Can you work these out from the model? Positions are in its coordinate system, mm. Coordinates: 2 decimals unless noted, no trailing zeros. Order: outer loops, then holes, each group sorted by start corner. A loop starts at its lowest first (then second) coordinate and runs counter-clockwise, first axis right, second up. Notation, with made-up numbers: (45, 8.25) -> (98, 8.25) arc R15 cw to (98, 14.25) -> close; hole circle Ø10 at (-32, 18.25). An arc over 180 degrees is marked (long way). Answer in a Markdown table with one row per item.
```python
from build123d import *

# Parameters (mm, degrees)
SKETCH1_W           = 50.8
SKETCH1_H           = 95.25
SKETCH1_R           = 2.413
BOSS_EXTRUDE1_DEPTH = 6.35
FILLET1_R           = 6.35
CHAMFER1_SIZE       = 2.54


with BuildPart() as part:
    # Sketch1 → Boss-Extrude1 (new body)
    with BuildSketch(Plane.XY):
        with Locations((25.4, 47.625)):
            Rectangle(SKETCH1_W, SKETCH1_H)
        with Locations((25.4, 69.85)):
            Circle(SKETCH1_R, mode=Mode.SUBTRACT)
        with Locations((25.4, 25.4)):
            Circle(SKETCH1_R, mode=Mode.SUBTRACT)
        with Locations((25.4, 57.15)):
            Circle(SKETCH1_R, mode=Mode.SUBTRACT)
        with Locations((25.4, 12.7)):
            Circle(SKETCH1_R, mode=Mode.SUBTRACT)
        with Locations((25.4, 38.1)):
            Circle(SKETCH1_R, mode=Mode.SUBTRACT)
        with Locations((25.4, 82.55)):
            Circle(SKETCH1_R, mode=Mode.SUBTRACT)
    extrude(amount=BOSS_EXTRUDE1_DEPTH)

    # Fillet1
    fillet1_edges = [part.edges().sort_by_distance(p)[0] for p in [
        (0, 95.25, 3.175),
        (50.8, 95.25, 3.175),
        (50.8, 0, 3.175),
        (0, 0, 3.175),
    ]]
    fillet(fillet1_edges, radius=FILLET1_R)

    # Chamfer1
    chamfer1_edges = [part.edges().sort_by_distance(p)[0] for p in [
        (22.987, 69.85, 6.35),
        (22.987, 25.4, 6.35),
        (22.987, 57.15, 6.35),
        (22.987, 12.7, 6.35),
        (22.987, 38.1, 6.35),
        (22.987, 82.55, 6.35),
    ]]
    chamfer(chamfer1_edges, length=CHAMFER1_SIZE)


solid = part.part
```
(1) Suppose I cut it at A-A (z = 2). Please give me the cut outline in (x, y), and give its area (3 significant figures).
Response values:
| item | result |
|---|---|
| outline | (0, 6.35) arc R6.35 ccw to (6.35, 0) -> (44.45, 0) arc R6.35 ccw to (50.8, 6.35) -> (50.8, 88.9) arc R6.35 ccw to (44.45, 95.25) -> (6.35, 95.25) arc R6.35 ccw to (0, 88.9) -> close; hole circle Ø4.83 at (25.4, 12.7); hole circle Ø4.83 at (25.4, 25.4); hole circle Ø4.83 at (25.4, 38.1); hole circle Ø4.83 at (25.4, 57.15); hole circle Ø4.83 at (25.4, 69.85); hole circle Ø4.83 at (25.4, 82.55) |
| area | 4,690 mm2 |
(2) Suppose I cut it at B-B (y = 12.7). Please give me the cut outline in (x, z).
Response values:
| item | result |
|---|---|
| outline | (0, 0) -> (22.99, 0) -> (22.99, 3.81) -> (20.45, 6.35) -> (0, 6.35) -> close; (27.81, 0) -> (50.8, 0) -> (50.8, 6.35) -> (30.35, 6.35) -> (27.81, 3.81) -> close |
(3) We'd pull the mould along Y, two halves only. Please class faces 1 (the flat face through (25, 48, 0)), 2 (the conical face through (25.07, 59.66, 3.93)), 3 (the conical face through (26.57, 80.3, 3.933)), 4 (the cylindrical face through (48.89, 1.81, 3.22)): +Y half, -Y half, draft (parallel to the pull), parting line (faces both ways), or undercut.
Response values:
| item | result |
|---|---|
| face 1 | draft |
| face 2 | undercut |
| face 3 | undercut |
| face 4 | -Y half |
(4) Will these pins go through, and if not, where does the flat tip stop? pin 1 Ø1.5 at (x, y) = (29, 23.5) entering from +Z; pin 2 Ø6.5 at (x, y) = (25.4, 12.7) entering from +Z.
Response values:
| item | result |
|---|---|
| pin 1 | z = 6.22 |
| pin 2 | z = 4.65 |
(5) Suppose I cut it at C-C (x = 25.4). Count the separate pieces of the cut face and the enclosed holes in it, and give its area (3 significant figures).
Response values:
| item | result |
|---|---|
| separate pieces | 7 |
| enclosed holes | 0 |
| area | 382 mm2 |
(6) I need wall thicknesses on line 1 (X direction, y = 55, z = 5.75); line 2 (X direction, y = 89, z = 2.5); line 3 (X direction, y = 10.5, z = 1). Which ranges of each line are inside material? Lowest first, please. Write a range as [from, to].
Response values:
| item | result |
|---|---|
| line 1 | [0, 21.62], [29.18, 50.8] |
| line 2 | [0, 50.8] |
| line 3 | [0, 24.41], [26.39, 50.8] |
